Geometry: final body of the model. Coordinates: model frame, mm. Face numbers are marked on the shaded views. A direction names the side the tool comes from. Coordinates: 2 decimals unless noted, no trailing zeros. Order: outer loops, then holes, each group sorted by start corner. A loop starts at its lowest first (then second) coordinate and runs counter-clockwise, first axis right, second up. Notation, with made-up numbers: M 16,-25.75 L 72,-25.75 A27 cw 72,-0.75 Z; hole C 20.25,-26 d7. An arc over 180 degrees is marked long. Use CSV: the item, a comma, the result in double quotes. Start each with the question number.
1. First-contact query: P1, Ø0.9, axis at x = -9.5, z = 0.5, coming from the -Y side; P2, Ø1.5, axis at y = -9, z = 0.5, coming from the +X side; P3, Ø4, axis at x = 1.5, y = 5, coming from the -Z side; P4, Ø0.9, axis at y = -9.5, z = 0.5, coming from the +X side. Flat tips, straight axial feed; report the tip coordinate or a pass-through.
2. Section query C-C on z = -1.15. Return the cut outline in (x, y).
3. Material intervals for line 1 (Y direction, x = 0, z = -0.6); line 2 (X direction, y = -0.25, z = 0.55); line 3 (Y direction, x = -2.25, z = 1), sorted ascending.
4. Set-up query: the marked faces 4, 5, 6 and 7. Return all of +Z, -Z, +X, -X, +Y, -Y with unobstructed straight access to the full face (end or side cutting, diameter ignored); none if empty.
5. Section query D-D on x = 10. Return the cut outline in (y, z).
6. Section query A-A on y = 0. Return the cut outline in (x, z), and give its area (3 significant figures).
7. Section query B-B on x = 4. Return the cut outline in (y, z).
8. Pull-direction query (X, two-part tool) for the marked faces 1, 2 and 3; classes: pulls with the +X half, pulls with the -X half, needs draft (parallel to the pull), parting line crosses it, or undercut.
Autodesk Inventor part; units mm, degrees
ref_plane "YZ Plane" through (0, 0, 0) normal (1, 0, 0) x (0, 1, 0)
ref_plane "XZ Plane" through (0, 0, 0) normal (0, 1, 0) x (-1, 0, 0)
ref_plane "XY Plane" through (0, 0, 0) normal (0, 0, 1) x (1, 0, 0)
sketch "Sketch1" plane through (0, 0, 0) normal (0, 0, 1) x (1, 0, 0)
  circle A0 centre (0, 0) radius 7.5
  line L0 (15, 5.6667) -> (12, 5.6667)
  line L1 (12, 5.6667) -> (12, 8.5)
  line L2 (12, -8.5) -> (12, -5.6667)
  line L3 (12, -5.6667) -> (15, -5.6667)
  line L4 (-8, -11.5) -> (-8, -8.5)
  line L5 (-8, -8.5) -> (-12, -8.5)
  line L6 (8, -11.5) -> (8, -8.5)
  line L7 (8, -8.5) -> (12, -8.5)
  line L8 (-15, -5.6667) -> (-12, -5.6667)
  line L9 (-12, -5.6667) -> (-12, -8.5)
  line L10 (-15, 5.6667) -> (-12, 5.6667)
  line L11 (-12, 5.6667) -> (-12, 8.5)
  line L12 (-8, 11.5) -> (-8, 8.5)
  line L13 (-8, 8.5) -> (-12, 8.5)
  line L14 (12, 8.5) -> (8, 8.5)
  line L15 (8, 8.5) -> (8, 11.5)
  line L16 (15, 5.6667) -> (15, -5.6667)
  line L17 (-8, 11.5) -> (8, 11.5)
  line L18 (-15, -5.6667) -> (-15, 5.6667)
  line L19 (8, -11.5) -> (-8, -11.5)
  line L20 (15, -5.1667) -> (15, 5.6667)
  line L21 (-20.9424, 0) -> (31.3224, 0) construction
  line L22 (0, 36) -> (0, -23) construction
  dimension "d0" = 15
  dimension "d3" = 3
  dimension "d5" = 3
  dimension "d6" = 3
  dimension "d16" = 3
  dimension "d18" = 24
  dimension "d19" = 16
  dimension "d21" = 17
  dimension "d22" = 11.3333
extrude "Extrusion1" add sketch "Sketch1" along normal mid plane 3
equation "\"d19\" = 0.666667 * d18"
equation "\"d22\" = 0.666667 * d21"
properties part number "Camera-Holder_Bearing-Ring-Middle-Right"
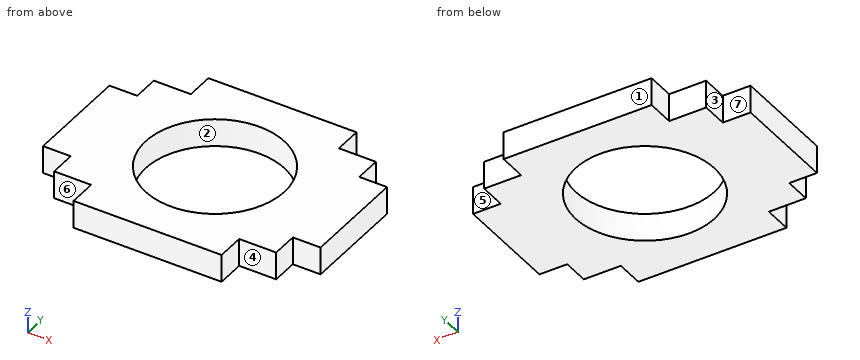
Results list:
1,P1,"stops at y = -8.5"
1,P2,"stops at x = 12"
1,P3,"passes through"
1,P4,"stops at x = 8"
2,outline,"M -15,-5.67 L -12,-5.67 L -12,-8.5 L -8,-8.5 L -8,-11.5 L 8,-11.5 L 8,-8.5 L 12,-8.5 L 12,-5.67 L 15,-5.67 L 15,5.67 L 12,5.67 L 12,8.5 L 8,8.5 L 8,11.5 L -8,11.5 L -8,8.5 L -12,8.5 L -12,5.67 L -15,5.67 Z; hole C 0,0 d15"
3,line 1,"y = -11.5 to -7.5, 7.5 to 11.5"
3,line 2,"x = -15 to -7.5, 7.5 to 15"
3,line 3,"y = -11.5 to -7.15, 7.15 to 11.5"
4,face 4,"+Z, -Z, +X, -Y"
4,face 5,"+Z, -Z, +X, +Y"
4,face 6,"+Z, -Z, -X, -Y"
4,face 7,"+Z, -Z, -X, +Y"
5,outline,"M -8.5,-1.5 L 8.5,-1.5 L 8.5,1.5 L -8.5,1.5 Z"
6,outline,"M -15,-1.5 L -7.5,-1.5 L -7.5,1.5 L -15,1.5 Z; M 7.5,-1.5 L 15,-1.5 L 15,1.5 L 7.5,1.5 Z"
6,area,"45.0 mm²"
7,outline,"M -11.5,-1.5 L -6.34,-1.5 L -6.34,1.5 L -11.5,1.5 Z; M 6.34,-1.5 L 11.5,-1.5 L 11.5,1.5 L 6.34,1.5 Z"
8,face 1,"needs draft"
8,face 2,"undercut"
8,face 3,"pulls with the -X half"
